Autodesk Inventor part; units mm, degrees
ref_plane "YZ Plane" through (0, 0, 0) normal (1, 0, 0) x (0, 1, 0)
ref_plane "XZ Plane" through (0, 0, 0) normal (0, 1, 0) x (-1, 0, 0)
ref_plane "XY Plane" through (0, 0, 0) normal (0, 0, 1) x (1, 0, 0)
sketch "Sketch1" plane through (0, 0, 0) normal (0, 0, 1) x (1, 0, 0)
  circle A0 centre (0, 0) radius 10
  line L0 (-57, -58) -> (42, -58)
  line L1 (42, -58) -> (54.739, -23)
  line L2 (54.739, -23) -> (52, -23)
  line L3 (52, -23) -> (52, -11)
  line L4 (52, -11) -> (55, -11)
  line L5 (55, -11) -> (55, 12)
  line L6 (-57, -58) -> (-57, -23)
  line L7 (-57, -23) -> (-51, -23)
  line L8 (-51, -23) -> (-51, -11)
  line L9 (-51, -11) -> (-57, -11)
  line L10 (-57, -11) -> (-57, 0)
  arc A1 (53.9189, 18.4865) -> (-57, 0) centre (0, 0) ccw
  arc A2 (55, 12) -> (53.9189, 18.4865) centre (35, 12) ccw
  dimension "d0" = 20
  dimension "d1" = 57
  dimension "d2" = 20
  dimension "d3" = 99
  dimension "d4" = 6
  dimension "d5" = 110
  dimension "d6" = 3
  dimension "d7" = 12
  dimension "d8" = 58
  dimension "d9" = 12
  dimension "d10" = 55
  dimension "d11" = 47
extrude "Extrusion1" add sketch "Sketch1" along normal blind 1.5
fillet "Fillet1" radius 0.5 4 edges at (52, -23, 0.75) (52, -11, 0.75) (-51, -11, 0.75) (-51, -23, 0.75)
fillet "Fillet2" radius 1 4 edges at (-57, -11, 0.75) (-57, -23, 0.75) (55, -11, 0.75) (54.739, -23, 0.75)
fillet "Fillet3" radius 5 2 edges at (42, -58, 0.75) (-57, -58, 0.75)
properties part number "NPT Flange Outer"
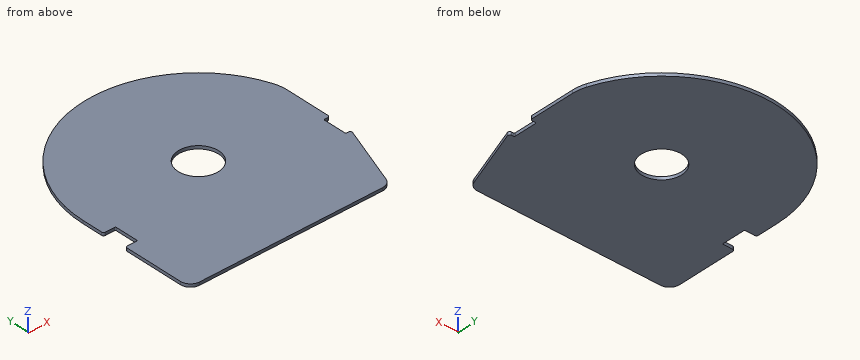
Read the model definition and answer for the solid it produces. Units are mm, in the model's axes. Give positions to 0.01 mm unless a question says otherwise; leave off trailing zeros. Loops run counter-clockwise (first coordinate to the right, second up) from the corner with the lowest first, then second, coordinate; pieces in that order, holes last. Notation, with made-up numbers: (-4, 70.25) -> (20, 70.25) arc R15 ccw to (20, 94.25) -> close; hole circle Ø10 at (88, 82). An arc over 180 degrees is marked (long way). Use a Markdown table: item, result.
Q1. Section C-C, the plane x = 31 is taken. Determine the outline of the cut face in (y, z).
Solved:
| item | result |
|---|---|
| outline | (-58, 0) -> (47.83, 0) -> (47.83, 1.5) -> (-58, 1.5) -> close |
Q2. Section A-A, the plane x = 0 is taken. Determine the outline of the cut face in (y, z), then the cut area to 4 significant figures.
Solved:
| item | result |
|---|---|
| outline | (-58, 0) -> (-10, 0) -> (-10, 1.5) -> (-58, 1.5) -> close; (10, 0) -> (57, 0) -> (57, 1.5) -> (10, 1.5) -> close |
| area | 142.5 mm^2 |
Q3. Section D-D, the plane x = 15 is taken. Determine the outline of the cut face in (y, z), then the cut area to 3 significant figures.
Solved:
| item | result |
|---|---|
| outline | (-58, 0) -> (54.99, 0) -> (54.99, 1.5) -> (-58, 1.5) -> close |
| area | 169 mm^2 |
Q4. Section B-B, the plane z = 0.75 is taken. Determine the outline of the cut face in (x, y).
Solved:
| item | result |
|---|---|
| outline | (-57, -53) arc R5 ccw to (-52, -58) -> (38.5, -58) arc R5 ccw to (43.2, -54.71) -> (54.25, -24.34) arc R1 ccw to (53.31, -23) -> (52.5, -23) arc R0.5 cw to (52, -22.5) -> (52, -11.5) arc R0.5 cw to (52.5, -11) -> (54, -11) arc R1 ccw to (55, -10) -> (55, 12) arc R20 ccw to (53.92, 18.49) arc R57 ccw to (-57, 0) -> (-57, -10) arc R1 ccw to (-56, -11) -> (-51.5, -11) arc R0.5 cw to (-51, -11.5) -> (-51, -22.5) arc R0.5 cw to (-51.5, -23) -> (-56, -23) arc R1 ccw to (-57, -24) -> close; hole circle Ø20 at (0, 0) |
Q5. This flat-tipped pin is pushed along its axis until it touches: pin 1 (0.8 mm diameter, centred on x = -54, z = 0.5, fed in from -Y). Where does it stop, or does it pass through?
Solved:
| item | result |
|---|---|
| pin 1 | stops at y = -57.74 |
Q6. Find the intervals of material crossed by line 1 along Y through (x, z) = (0, 1.25); line 2 along X through (y, z) = (-4.5, 0.95); line 3 along X through (y, z) = (7, 1.2), in increasing order.
Solved:
| item | result |
|---|---|
| line 1 | y = -58 to -10, 10 to 57 |
| line 2 | x = -57 to -8.93, 8.93 to 55 |
| line 3 | x = -56.57 to -7.14, 7.14 to 55 |
